Geometry check sheet. Reference: the model listing, model coordinates, mm. A direction names the side the tool comes from. Round coordinates to 2 decimals unless told otherwise and drop trailing zeros. Write each loop counter-clockwise with the first axis right and the second up, starting at its lowest first coordinate (ties: lowest second). Pieces come first, ordered by that corner, then holes. Notation, with made-up numbers: (38, 1.5) -> (51, 1.5) arc R19 ccw to (51, 21.5) -> close; hole circle Ø11 at (-5, 73). An arc over 180 degrees is marked (long way). Return JSON: item names as keys, results as strings. Group by question number.
from build123d import *

# Parameters (mm, degrees)
SKETCH1_R           = 1.75
SKETCH1_R_2         = 10.075
BOSS_EXTRUDE1_DEPTH = 5
CUT_EXTRUDE1_START  = -5
SKETCH2_W           = 4.2
SKETCH2_H           = 26.15
CUT_EXTRUDE1_DEPTH  = 5
SKETCH3_R           = 16.075
BOSS_EXTRUDE2_DEPTH = 0.5
BOSS_EXTRUDE3_DEPTH = 5.5
SKETCH5_R           = 3.025
CUT_EXTRUDE2_DEPTH  = 2.05
CUT_EXTRUDE3_START  = -3
CUT_EXTRUDE3_DEPTH  = 3


with BuildPart() as part:
    # Sketch1 → Boss-Extrude1 (new body)
    with BuildSketch(Plane(origin=(0, 0, 0), x_dir=(0, 0, -1), z_dir=(1, 0, 0))):
        with BuildLine():
            Line((4.75, 15.357184801), (4.75, 18.575))
            ThreePointArc((4.75, 18.575), (0, 23.325), (-4.75, 18.575))
            Line((-4.75, 18.575), (-4.75, 15.357184801))
            ThreePointArc((-4.75, 15.357184801), (-16.075, 0), (-4.75, -15.357184801))
            Line((-4.75, -15.357184801), (-4.75, -18.575))
            ThreePointArc((-4.75, -18.575), (0, -23.325), (4.75, -18.575))
            Line((4.75, -18.575), (4.75, -15.357184801))
            ThreePointArc((4.75, -15.357184801), (16.075, 0), (4.75, 15.357184801))
        make_face()
        with Locations((0, 18.575)):
            Circle(SKETCH1_R, mode=Mode.SUBTRACT)
        Circle(SKETCH1_R_2, mode=Mode.SUBTRACT)
        with Locations(Location((0, -18.575, 0), (0, 0, 180))):
            Circle(SKETCH1_R, mode=Mode.SUBTRACT)
    extrude(amount=BOSS_EXTRUDE1_DEPTH)

    # Sketch2 → Cut-Extrude1 (cut)
    with BuildSketch(Plane.ZY.offset(CUT_EXTRUDE1_START)):
        Rectangle(SKETCH2_W, SKETCH2_H)
    extrude(amount=CUT_EXTRUDE1_DEPTH, mode=Mode.SUBTRACT)

    # Sketch3 → Boss-Extrude2 (add)
    with BuildSketch(Plane(origin=(5, 0, 0), x_dir=(0, 0, -1), z_dir=(1, 0, 0))):
        with Locations(Location((0, 0, 0), (0, 0, 107.186915706))):
            Circle(SKETCH3_R)
        with BuildLine():
            Line((-2.1, 13.075), (-2.1, 9.85371123))
            ThreePointArc((-2.1, 9.85371123), (-10.075, 0), (-2.1, -9.85371123))
            Line((-2.1, -9.85371123), (-2.1, -13.075))
            Line((-2.1, -13.075), (2.1, -13.075))
            Line((2.1, -13.075), (2.1, -9.85371123))
            ThreePointArc((2.1, -9.85371123), (10.075, 0), (2.1, 9.85371123))
            Line((2.1, 9.85371123), (2.1, 13.075))
            Line((2.1, 13.075), (-2.1, 13.075))
        make_face(mode=Mode.SUBTRACT)
    extrude(amount=BOSS_EXTRUDE2_DEPTH)

    # Sketch4 → Boss-Extrude3 (add)
    with BuildSketch(Plane.ZY):
        with BuildLine():
            Line((-13.5, -4.5), (-9.014190202, -4.5))
            ThreePointArc((-9.014190202, -4.5), (-10.075, 0), (-9.014190202, 4.5))
            Line((-9.014190202, 4.5), (-13.5, 4.5))
            ThreePointArc((-13.5, 4.5), (-18, 0), (-13.5, -4.5))
        make_face()
        with BuildLine():
            Line((13.5, 4.5), (9.014190202, 4.5))
            ThreePointArc((9.014190202, 4.5), (10.075, 0), (9.014190202, -4.5))
            Line((9.014190202, -4.5), (13.5, -4.5))
            ThreePointArc((13.5, -4.5), (18, 0), (13.5, 4.5))
        make_face()
    extrude(amount=-BOSS_EXTRUDE3_DEPTH)

    # Sketch5 → Cut-Extrude2 (cut)
    with BuildSketch(Plane(origin=(5.5, 0, 0), x_dir=(0, 0, -1), z_dir=(1, 0, 0))):
        with Locations((-13.5, 0)):
            Circle(SKETCH5_R)
        with Locations((13.5, 0)):
            Circle(SKETCH5_R)
    extrude(amount=-CUT_EXTRUDE2_DEPTH, mode=Mode.SUBTRACT)

    # Sketch6 → Cut-Extrude3 (cut)
    with BuildSketch(Plane(origin=(5, 0, 0), x_dir=(0, 0, -1), z_dir=(1, 0, 0)).offset(CUT_EXTRUDE3_START)):
        with BuildLine():
            Line((4.75, 15.357184801), (4.75, 18.575))
            ThreePointArc((4.75, 18.575), (0, 23.325), (-4.75, 18.575))
            Line((-4.75, 18.575), (-4.75, 15.357184801))
            ThreePointArc((-4.75, 15.357184801), (0, 16.075), (4.75, 15.357184801))
        make_face()
        with BuildLine():
            Line((-4.75, -15.357184801), (-4.75, -18.575))
            ThreePointArc((-4.75, -18.575), (0, -23.325), (4.75, -18.575))
            Line((4.75, -18.575), (4.75, -15.357184801))
            ThreePointArc((4.75, -15.357184801), (0, -16.075), (-4.75, -15.357184801))
        make_face()
    extrude(amount=CUT_EXTRUDE3_DEPTH, mode=Mode.SUBTRACT)


solid = part.part
1) Sectioned sample at D-D on z = 6.5. Enter the section's corners in (x, y), and give its area (3 significant figures).
2) Go/stop test with flat-tipped pins: P1, Ø3, axis at x = 4, y = 7.5, coming from the -Z side; P2, Ø1.6, axis at x = 0.5, y = 18, coming from the +Z side; P3, Ø1.5, axis at x = 2, y = -9, coming from the -Z side. Record where each tip stops, or that it passes through.
3) Sectioned sample at A-A on x = 2.75. Enter the section's corners in (y, z) (3 decimals).
4) Tool access check on faces 1 (the face through (1, 17, 4.75)), 2 (the face through (3.45, 0, 14)), 3 (the face through (1, -17, -4.75)). Record the directions out of +Z, -Z, +X, -X, +Y, -Y that give a thin tool (end or side, any length) a straight path to the whole face; none if there is none.
5) Sectioned sample at B-B on z = 0. Enter the section's corners in (x, y) (3 decimals).
6) Material ranges on probe 1 along Y at (x, z) = (0.5, 0) (3 decimals); probe 2 along Z at (x, y) = (4.1, 2); probe 3 along Y at (x, z) = (1.5, -1) (3 decimals), recorded low to high. Write a range as [from, to].
7) Sectioned sample at C-C on y = 0. Enter the section's corners in (x, z) (3 decimals).
8) Mould release check, pull along Z, two halves, no side actions. Record for faces 4 (the face through (5.5, 9, -5)), 5 (the face through (3, 0, -18)), 6 (the face through (3, -11, 2.1)): +Z half, -Z half, draft (parallel to the pull), parting line (faces both ways), or undercut.
Evaluation:
{
 "1": {"outline": "(0, -14.7) -> (5.5, -14.7) -> (5.5, -7.7) -> (0, -7.7) -> close; (0, 7.7) -> (5.5, 7.7) -> (5.5, 14.7) -> (0, 14.7) -> close", "area": "77.0 mm2"},
 "2": {"P1": "stops at z = -14.91", "P2": "stops at z = 4.75", "P3": "stops at z = -13.8"},
 "3": {"outline": "(-3.995, -15.571) arc R4.5 ccw to (3.995, -15.571) arc R16.075 ccw to (3.995, 15.571) arc R4.5 ccw to (-3.995, 15.571) arc R16.075 ccw to start; hole (-13.075, -2.1) -> (-9.854, -2.1) arc R10.075 ccw to (9.854, -2.1) -> (13.075, -2.1) -> (13.075, 2.1) -> (9.854, 2.1) arc R10.075 ccw to (-9.854, 2.1) -> (-13.075, 2.1) -> close"},
 "4": {"face 1": "+Z, +X, -X, +Y", "face 2": "+X", "face 3": "-Z, +X, -X, -Y"},
 "5": {"outline": "(0, -23.325) -> (2, -23.325) -> (2, -20.325) -> (0, -20.325) -> close; (0, -16.825) -> (2, -16.825) -> (2, -16.075) -> (5.5, -16.075) -> (5.5, -13.075) -> (0, -13.075) -> close; (0, 13.075) -> (5.5, 13.075) -> (5.5, 16.075) -> (2, 16.075) -> (2, 16.825) -> (0, 16.825) -> close; (0, 20.325) -> (2, 20.325) -> (2, 23.325) -> (0, 23.325) -> close"},
 "6": {"probe 1": "y = [-23.325, -20.325], [-16.825, -13.075], [13.075, 16.825], [20.325, 23.325]", "probe 2": "z = [-17.53, -15.77], [-11.23, -9.87], [9.87, 11.23], [15.77, 17.53]", "probe 3": "y = [-23.219, -20.011], [-17.139, -13.075], [13.075, 17.139], [20.011, 23.219]"},
 "7": {"outline": "(0, -18) -> (5.5, -18) -> (5.5, -16.525) -> (3.45, -16.525) -> (3.45, -10.475) -> (5.5, -10.475) -> (5.5, -10.075) -> (0, -10.075) -> close; (0, 10.075) -> (5.5, 10.075) -> (5.5, 10.475) -> (3.45, 10.475) -> (3.45, 16.525) -> (5.5, 16.525) -> (5.5, 18) -> (0, 18) -> close"},
 "8": {"face 4": "draft", "face 5": "-Z half", "face 6": "undercut"}
}
